Work out the finished part from the listing and answer in its coordinate system (mm). A direction names the side the tool comes from. Round coordinates to 2 decimals unless told otherwise and drop trailing zeros. Loops run counter-clockwise (first coordinate to the right, second up) from the corner with the lowest first, then second, coordinate; pieces in that order, holes last. Notation, with made-up numbers: (-26, 27) -> (-5, 27) arc R21 cw to (-5, 57) -> close; hole circle Ø5 at (21.25, -11). An arc over 180 degrees is marked (long way). Use CSV: the item, a comma, the result in double quotes. Start each with the question number.
Autodesk Fusion 360 part; units mm, degrees
sketch "Sketch1" plane through (0, 0, 0) normal (0, 0, 1) x (1, 0, 0)
  line L0 (0, 0) -> (110, 0)
  line L1 (110, 0) -> (110, 75)
  line L2 (110, 75) -> (0, 75)
  line L3 (0, 75) -> (0, 0)
  dimension "d1" = 110
  dimension "d2" = 75
extrude "Extrude1" add sketch "Sketch1" along normal blind 2
sketch "Screws" plane through (0, 0, 2) normal (0, 0, 1) x (1, 0, 0)
  line L0 (107, 72) -> (107, 3)
  line L1 (3, 3) -> (3, 72)
  line L2 (3, 72) -> (107, 72)
  line L3 (107, 3) -> (3, 3)
  line L4 (110, 75) -> (0, 75)
  line L5 (0, 0) -> (110, 0)
  line L6 (110, 0) -> (110, 75)
  line L7 (0, 75) -> (0, 0)
  line L8 (1.5, 65) -> (1.5, 10)
  line L9 (108.5, 65) -> (1.5, 65)
  line L10 (1.5, 10) -> (108.5, 10)
  line L11 (108.5, 10) -> (108.5, 65)
  dimension "d10" = 107
  dimension "d12" = 10
  dimension "d13" = 65
hole "Hole1" at (1.5, 10, 2) at (1.5, 65, 2) at (108.5, 65, 2) at (108.5, 10, 2) direction (0, 0, -1) diameter 2 depth 19 tip angle 180
sketch "screw holes" plane through (0, 0, 2) normal (0, 0, 1) x (1, 0, 0)
  line L0 (3, 3) -> (3, 72)
  line L1 (3, 72) -> (107, 72)
  line L2 (107, 72) -> (107, 3)
  line L3 (107, 3) -> (3, 3)
  line L4 (110, 75) -> (0, 75)
  line L5 (0, 0) -> (110, 0)
  line L6 (110, 0) -> (110, 75)
  line L7 (0, 75) -> (0, 0)
  line L8 (1.5, 15) -> (108.5, 15)
  line L9 (108.5, 15) -> (108.5, 65)
  line L10 (1.5, 65) -> (1.5, 15)
  line L11 (108.5, 65) -> (1.5, 65)
extrude "Extrude2" add sketch "screw holes" along normal blind 2 contours L0 L2 L3 L8 | L0 L2 L8 L11 | L0 L1 L2 L11
sketch "Sketch4" plane through (0, 0, 4) normal (0, 0, 1) x (-1, 0, 0)
  line L0 (-107, -3) -> (-107, -72)
  line L1 (-107, -72) -> (-3, -72)
  line L2 (-3, -72) -> (-3, -3)
  line L3 (-3, -3) -> (-107, -3)
  line L4 (-34, -7) -> (-60, -7)
  line L5 (-60, -7) -> (-60, -21)
  line L6 (-60, -21) -> (-34, -21)
  line L7 (-34, -21) -> (-34, -7)
  point P0 (-34, -7)
  dimension "d14" = 7
  dimension "d15" = 34
  dimension "d16" = 60
  dimension "d17" = 21
extrude "Extrude3" cut sketch "Sketch4" against normal blind 5 contours L4 L5 L6 L7
fillet "Fillet1" radius 2 1 edges at (55, 72, 4)
fillet "Fillet1" radius 2 1 edges at (110, 75, 1)
fillet "Fillet1" radius 2 1 edges at (110, 0, 1)
fillet "Fillet1" radius 2 1 edges at (0, 0, 1)
fillet "Fillet1" radius 2 1 edges at (0, 75, 1)
fillet "Fillet1" radius 2 1 edges at (60, 21, 2)
fillet "Fillet1" radius 2 1 edges at (60, 7, 2)
fillet "Fillet1" radius 2 1 edges at (34, 7, 2)
fillet "Fillet1" radius 2 1 edges at (34, 21, 2)
equation "d13 = 75 mm - d12"
Q1. Which of the six approach directions +Z, -Z, +X, -X, +Y, -Y give full straight-line access (tool end or side, diameter ignored) to faces 4 (the flat face through (56, 3, 3)), 5 (the flat face through (47, 21, 2)), 6 (the flat face through (3, 37, 3)), 7 (the cylindrical face through (109.43, 74.4, 1.01))?
Q2. Each of these flat-tipped pins is pushed along its axis until it touches: pin 1 (0.6 mm diameter, centred on y = 33, z = 3, fed in from +X); pin 2 (1.2 mm diameter, centred on x = 44.5, z = 3, fed in from -Y); pin 3 (1.8 mm diameter, centred on x = 108.5, y = 65, fed in from +Z); pin 4 (2.5 mm diameter, centred on x = 1.5, y = 65, fed in from +Z). Where does it stop, or does it pass through?
Q3. Section C-C, the plane z = 1.3 is taken. Write down the section's boundary in (x, y), and give its area (3 significant figures).
Q4. Section B-B, the plane y = 12.5 is taken. Write down the section's boundary in (x, z).
Q5. For a pull along Y with two mould halves and no side action, classify faces 1 (the flat face through (54, 0, 1)), 2 (the flat face through (60, 14, 2)), 3 (the flat face through (0, 38, 1)) as pulls with the +Y half, pulls with the -Y half, needs draft (parallel to the pull), parting line crosses it, or undercut.
Q6. Straight lines are drawn through the part: line 1 (X direction, y = 65, z = 0.75); line 2 (X direction, y = 10, z = 0.4); line 3 (X direction, y = 16, z = 2.1). For each, find the intervals that lie inside material, in ascending order. Write a range as from..to.
Q7. Section D-D, the plane y = 54 is taken. Write down the section's boundary in (x, z).
Report:
1,face 4,"+Z, +X, -X, -Y"
1,face 5,"+Z, -Z"
1,face 6,"+Z, -X, +Y, -Y"
1,face 7,"+Z, -Z, +X, +Y"
2,pin 1,"stops at x = 107"
2,pin 2,"stops at y = 3"
2,pin 3,"passes through"
2,pin 4,"stops at z = 2"
3,outline,"(0, 2) arc R2 ccw to (2, 0) -> (108, 0) arc R2 ccw to (110, 2) -> (110, 73) arc R2 ccw to (108, 75) -> (2, 75) arc R2 ccw to (0, 73) -> close; hole circle Ø2 at (1.5, 10); hole circle Ø2 at (1.5, 65); hole (34, 9) arc R2 ccw to (36, 7) -> (58, 7) arc R2 ccw to (60, 9) -> (60, 19) arc R2 ccw to (58, 21) -> (36, 21) arc R2 ccw to (34, 19) -> close; hole circle Ø2 at (108.5, 10); hole circle Ø2 at (108.5, 65)"
3,area,"7,870 mm²"
4,outline,"(0, 0) -> (34, 0) -> (34, 4) -> (3, 4) -> (3, 2) -> (0, 2) -> close; (60, 0) -> (110, 0) -> (110, 2) -> (107, 2) -> (107, 4) -> (60, 4) -> close"
5,face 1,"pulls with the -Y half"
5,face 2,"undercut"
5,face 3,"needs draft"
6,line 1,"x = 0..0.5, 2.5..107.5, 109.5..110"
6,line 2,"x = 0..0.5, 2.5..34, 60..107.5, 109.5..110"
6,line 3,"x = 3..34, 60..107"
7,outline,"(0, 0) -> (110, 0) -> (110, 2) -> (107, 2) -> (107, 4) -> (3, 4) -> (3, 2) -> (0, 2) -> close"
